Here's how the part is built. I have some questions about the finished solid (model axes, mm). A direction names the side the tool comes from. Coordinates: 2 decimals unless noted, no trailing zeros. Order: outer loops, then holes, each group sorted by start corner. A loop starts at its lowest first (then second) coordinate and runs counter-clockwise, first axis right, second up. Notation, with made-up numbers: (67.5, 20) - (106.5, 20) arc R15 ccw to (106.5, 39) - close; hole circle Ø6 at (9, 15). An arc over 180 degrees is marked (long way). Answer as CSV lines item,"result". Start each with the question number.
Q1. Suppose I cut it at C-C (y = -2). Please give me the cut outline in (x, z), then the cut area to 3 significant figures.
Q2. Suppose I cut it at A-A (z = -9.5). Please give me the cut outline in (x, y), then the cut area to 3 significant figures.
Q3. For pin 1 Ø3 at (x, y) = (28.5, -1.5) entering from -Z; pin 2 Ø10 at (x, z) = (38, -31) entering from +Y; pin 3 Ø3 at (x, y) = (23, -1) entering from +Z, each with a flat end and sliding along its axis, tell me the tip position at first contact or that it passes through.
Q4. Suppose I cut it at B-B (x = 6). Please give me the cut outline in (y, z).
Q5. Suppose I cut it at D-D (z = 2). Please give me the cut outline in (x, y).
Q6. I need wall thicknesses on line 1 (Z direction, x = 22.5, y = -2.25); line 2 (X direction, y = 2.75, z = -31.5); line 3 (X direction, y = 3, z = 14). Which ranges of each line are inside material? Lowest first, please.
Q7. For faces 1 (the face through (-9, -3, 0)), 2 (the face through (40, -3, -20)), 3 (the face through (1.846, -3.549, -0.245)), 4 (the face through (40, 3, -20)), 5 (the face through (33, 0, -35)), which set-ups out of +Z, -Z, +X, -X, +Y, -Y let a thin tool reach every point of the face, with its end or its side?
Q8. Thinking about a two-plate mould opening in X: for faces 6 (the face through (61.99, 0.04, -59.65)), 7 (the face through (-11, 3, 0)), 8 (the face through (-18, -2, 0)), 9 (the face through (29.99, 0.04, -10.35)), which applies, released by +X, released by -X, zero draft, split by the parting line, or undercut?
from build123d import *

# Parameters (mm, degrees)
BOSS_EXTRUDE4_DEPTH      = 3
BOSS_EXTRUDE5_DEPTH      = 10
BOSS_EXTRUDE5_DEPTH_BACK = 25
SKETCH10_R               = 4
FILLET4_R                = 10
FILLET5_R                = 5


with BuildPart() as part:
    # Sketch9 → Boss-Extrude4 (new, symmetric)
    with BuildSketch(Plane(origin=(0, 0, 0), x_dir=(1, 0, 0), z_dir=(0, 1, 0))):
        Polygon((0, -7.5), (65, -7.5), (65, 62.5), (33, 62.5), (33, 7.5), (0, 7.5), (0, 5), (-20, 5), (-20, -5), (0, -5), align=None)
    extrude(amount=BOSS_EXTRUDE4_DEPTH, both=True)

    # Sketch10 → Boss-Extrude5 (add, two sides: drawn at the far end of the back side and taken through both)
    with BuildSketch(Plane.XY.offset(7.5).offset(-BOSS_EXTRUDE5_DEPTH_BACK)):
        Circle(SKETCH10_R)
    extrude(amount=BOSS_EXTRUDE5_DEPTH + BOSS_EXTRUDE5_DEPTH_BACK)

    # Fillet4
    fillet4_edges = [part.edges().sort_by_distance(p)[0] for p in [
        (33, 0, -7.5),
        (33, 0, -62.5),
        (65, 0, -62.5),
        (65, 0, 7.5),
    ]]
    fillet(fillet4_edges, radius=FILLET4_R)

    # Fillet5
    fillet5_edges = [part.edges().sort_by_distance(p)[0] for p in [
        (-20, -3, 0),
    ]]
    fillet(fillet5_edges, radius=FILLET5_R)


solid = part.part
Here are the results:
1,outline,"(-18, -5) - (-3.46, -5) - (-3.46, -17.5) - (3.46, -17.5) - (3.46, -7.5) - (23, -7.5) arc R10 cw to (33, -17.5) - (33, -52.5) arc R10 ccw to (43, -62.5) - (55, -62.5) arc R10 ccw to (65, -52.5) - (65, -2.5) arc R10 ccw to (55, 7.5) - (3.46, 7.5) - (3.46, 17.5) - (-3.46, 17.5) - (-3.46, 5) - (-18, 5) - close"
1,area,"3,030 mm²"
2,outline,"circle Ø8 at (0, 0); (29, -3) - (65, -3) - (65, 3) - (29, 3) - close"
2,area,"266 mm²"
3,pin 1,"stops at z = -10.36"
3,pin 2,"stops at y = 3"
3,pin 3,"stops at z = 7.5"
4,outline,"(-3, -7.5) - (3, -7.5) - (3, 7.5) - (-3, 7.5) - close"
5,outline,"(-20, 2) arc R5 ccw to (-15, -3) - (-2.65, -3) arc R4 ccw to (2.65, -3) - (63.93, -3) - (63.93, 3) - (2.65, 3) arc R4 ccw to (-2.65, 3) - (-20, 3) - close"
6,line 1,"z = -7.5 to 7.5"
6,line 2,"x = 33 to 65"
6,line 3,"x = -2.65 to 2.65"
7,face 1,"+Z, -Z, -X, -Y"
7,face 2,"+Z, -Z, +X, -Y"
7,face 3,"none"
7,face 4,"+Z, -Z, +X, +Y"
7,face 5,"-Z, -X, +Y, -Y"
8,face 6,"released by +X"
8,face 7,"zero draft"
8,face 8,"released by -X"
8,face 9,"undercut"
